from build123d import *

# Parameters (mm, degrees)
SKETCH1_W                = 100
SKETCH1_H                = 140
SKETCH1_R                = 23.49
BOSS_EXTRUDE1_DEPTH      = 13
M8_CLEARANCE_HOLE1_D     = 8.2
M8_CLEARANCE_HOLE1_DEPTH = 19.75
M8_CLEARANCE_HOLE1_TIP   = 2.463528538


with BuildPart() as part:
    # Sketch1 → Boss-Extrude1 (new body)
    with BuildSketch(Plane.XY):
        Rectangle(SKETCH1_W, SKETCH1_H)
        with Locations(Location((0, 0, 0), (0, 0, 180))):
            Circle(SKETCH1_R, mode=Mode.SUBTRACT)
    extrude(amount=BOSS_EXTRUDE1_DEPTH)

    # M8 Clearance Hole1
    with Locations(Plane(origin=(-30, 20, 13), x_dir=(1, 0, 0), z_dir=(0, 0, 1))):
        with Locations((0, 0), (60, 0), (60, -40), (0, -40)):
            Hole(M8_CLEARANCE_HOLE1_D / 2, depth=M8_CLEARANCE_HOLE1_DEPTH)
            with Locations((0, 0, -(M8_CLEARANCE_HOLE1_DEPTH + M8_CLEARANCE_HOLE1_TIP / 2))):  # 118° drill point
                Cone(0, M8_CLEARANCE_HOLE1_D / 2, M8_CLEARANCE_HOLE1_TIP, mode=Mode.SUBTRACT)


solid = part.part
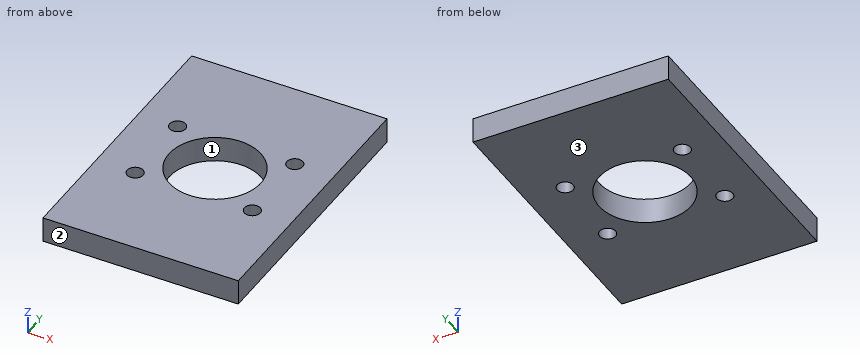
Can you work these out from the model? Positions are in its coordinate system, mm. Face numbers are marked on the shaded views. Give positions to 0.01 mm unless a question says otherwise; leave off trailing zeros. Loops run counter-clockwise (first coordinate to the right, second up) from the corner with the lowest first, then second, coordinate; pieces in that order, holes last. Notation, with made-up numbers: M -28,32.5 L 4,32.5 A35 ccw 4,64.5 Z; hole C 43,56.25 d6. An arc over 180 degrees is marked long. One line per item, written item: value. Start each with the question number.
1) Thinking about a two-plate mould opening in Y: for the marked faces 1, 2 and 3, which applies, +Y half, -Y half, draft (parallel to the pull), parting line (faces both ways), or undercut?
2) If we section it at B-B, the plane y = 0: Write out the boundary of the cut face in (x, z).
3) I'm going to push a flat-ended pin straight in: pin 1 (8 mm diameter, centred on x = -37.5, y = -54, fed in from -Z). Where does the tip first touch, or does it pass through?
4) If we section it at D-D, the plane x = 0: Write out the boundary of the cut face in (y, z).
5) If I drill on line 1 (Y direction, x = -30, z = 6.5); line 2 (X direction, y = -19, z = 6); line 3 (Y direction, x = 12.5, z = 4.75), over which ranges is the centre line in solid material (lowest first)? Write a range as [from, to].
6) If we section it at A-A, the plane x = 30: Write out the boundary of the cut face in (y, z).
7) If we section it at C-C, the plane z = 7.75: Write out the boundary of the cut face in (x, y).
Completed:
1. face 1: undercut
1. face 2: -Y half
1. face 3: draft
2. outline: M -50,0 L -23.49,0 L -23.49,13 L -50,13 Z; M 23.49,0 L 50,0 L 50,13 L 23.49,13 Z
3. pin 1: stops at z = 0
4. outline: M -70,0 L -23.49,0 L -23.49,13 L -70,13 Z; M 23.49,0 L 70,0 L 70,13 L 23.49,13 Z
5. line 1: y = [-70, -24.1], [-15.9, 15.9], [24.1, 70]
5. line 2: x = [-50, -33.98], [-26.02, -13.81], [13.81, 26.02], [33.98, 50]
5. line 3: y = [-70, -19.89], [19.89, 70]
6. outline: M -70,0 L -24.1,0 L -24.1,13 L -70,13 Z; M -15.9,0 L 15.9,0 L 15.9,13 L -15.9,13 Z; M 24.1,0 L 70,0 L 70,13 L 24.1,13 Z
7. outline: M -50,-70 L 50,-70 L 50,70 L -50,70 Z; hole C -30,-20 d8.2; hole C -30,20 d8.2; hole C 0,0 d46.98; hole C 30,-20 d8.2; hole C 30,20 d8.2
